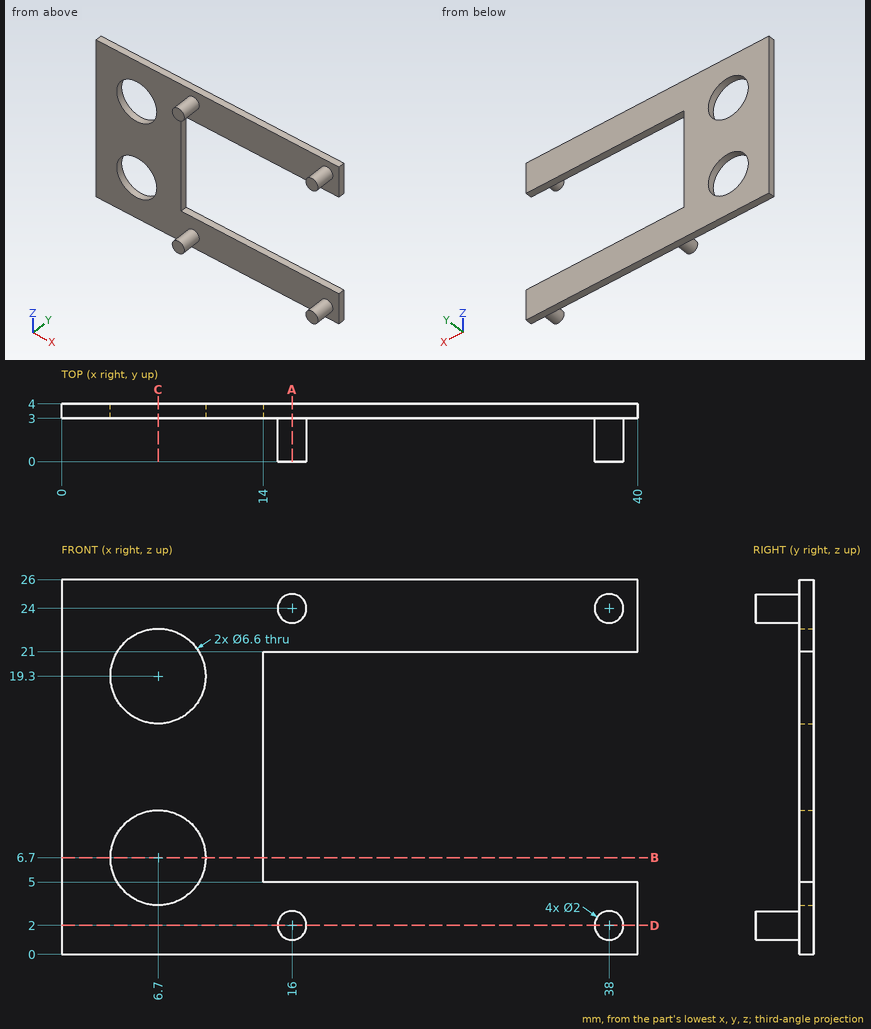
Verification items for this drawing (mm, ordinates from the low corner). Coordinates: 2 decimals unless noted, no trailing zeros. Loops run counter-clockwise (first coordinate to the right, second up) from the corner with the lowest first, then second, coordinate; pieces in that order, holes last. Notation, with made-up numbers: (2, -35.75) - (15, -35.75) arc R28 ccw to (15, -0.75) - close; hole circle Ø1 at (48, -17.5). An arc over 180 degrees is marked (long way). Answer as a JSON object with one key per item and string values.
(1) Cross-section at B-B, the plane z = 6.7. Record the boundary of the cut face in (x, y).
Response:
{"outline": "(0, 3) - (3.4, 3) - (3.4, 4) - (0, 4) - close; (10, 3) - (14, 3) - (14, 4) - (10, 4) - close"}
(2) Cross-section at C-C, the plane x = 6.7. Record the boundary of the cut face in (y, z), then the cut area to 3 significant figures.
Response:
{"outline": "(3, 0) - (4, 0) - (4, 3.4) - (3, 3.4) - close; (3, 10) - (4, 10) - (4, 16) - (3, 16) - close; (3, 22.6) - (4, 22.6) - (4, 26) - (3, 26) - close", "area": "12.8 mm²"}
(3) Go/stop test with a flat-tipped pin: pin 1 Ø13 at (x, z) = (12.5, 11.5) entering from -Y. Record where the tip stops, or that it passes through.
Response:
{"pin 1": "stops at y = 3"}
(4) Cross-section at A-A, the plane x = 16. Record the boundary of the cut face in (y, z), then the cut area to 3 significant figures.
Response:
{"outline": "(0, 1) - (3, 1) - (3, 0) - (4, 0) - (4, 5) - (3, 5) - (3, 3) - (0, 3) - close; (0, 23) - (3, 23) - (3, 21) - (4, 21) - (4, 26) - (3, 26) - (3, 25) - (0, 25) - close", "area": "22.0 mm²"}
(5) Scan lines: line 1 along Z through (x, y) = (6.7, 3.35); line 2 along Z through (x, y) = (24, 3.4); line 3 along Z through (x, y) = (7.5, 3.45). Record each from-to range of solid material in increasing order.
Response:
{"line 1": "z = 0 to 3.4, 10 to 16, 22.6 to 26", "line 2": "z = 0 to 5, 21 to 26", "line 3": "z = 0 to 3.5, 9.9 to 16.1, 22.5 to 26"}
(6) Cross-section at D-D, the plane z = 2. Record the boundary of the cut face in (x, y).
Response:
{"outline": "(0, 3) - (15, 3) - (15, 0) - (17, 0) - (17, 3) - (37, 3) - (37, 0) - (39, 0) - (39, 3) - (40, 3) - (40, 4) - (0, 4) - close"}
